Verification items for the finished model (mm, model axes). Face numbers are marked on the shaded views. A direction names the side the tool comes from. Round coordinates to 2 decimals unless told otherwise and drop trailing zeros. Write each loop counter-clockwise with the first axis right and the second up, starting at its lowest first coordinate (ties: lowest second). Pieces come first, ordered by that corner, then holes. Notation, with made-up numbers: M 63.5,88.5 L 106.5,88.5 A13 cw 106.5,103.5 Z; hole C -34.75,24.5 d4. An arc over 180 degrees is marked long. One line per question, with ' | ' between items. Start each with the question number.
Q1. Cross-section at A-A (y = 0). Record the boundary of the cut face in (x, z).
Q2. Tool access check on the marked faces 5 and 6. Record the directions out of +Z, -Z, +X, -X, +Y, -Y that give a thin tool (end or side, any length) a straight path to the whole face; none if there is none.
Q3. Thickness scan on line 1 along Y through (x, z) = (0, -0.65); line 2 along Y through (x, z) = (0, 4.75). Record the ranges inside material, lowest first. Write a range as from..to.
Q4. Cross-section at C-C (z = 9.5). Record the boundary of the cut face in (x, y).
Q5. Release check for a two-part mould opening along Y. For the marked faces 1, 2, 3 and 4 record: released by +Y, released by -Y, zero draft, split by the parting line, or undercut.
Q6. Gauge pin test, flat ends, axial feed: pin 1 (1.5 mm diameter, centred on y = 5.5, z = 0.5, fed in from -X); pin 2 (4 mm diameter, centred on x = -12.5, z = 8.5, fed in from -Y); pin 3 (4 mm diameter, centred on x = -9, z = 2, fed in from +Y); pin 4 (20 mm diameter, centred on x = 0, y = -3, fed in from +Z). Record the tip position at first contact, or that the pin passes through.
from build123d import *

# Parameters (mm, degrees)
F0_R     = 26.15
F1_DEPTH = 13.4
F2_R     = 12.6
F3_DEPTH = 7.4
F4_R     = 8.5
F5_DEPTH = 6
F6_R     = 13.5
F6_R_2   = 8.5
F7_DEPTH = 1
F8_SIZE  = 1


with BuildPart() as f1:
    # F0 (on Top) → F1 (new body)
    with BuildSketch(Plane.XY):
        Circle(F0_R)
    extrude(amount=F1_DEPTH)

    # F2 (on face) → F3 (cut)
    with BuildSketch(Plane.XY.offset(13.4)):
        Circle(F2_R)
    extrude(amount=-F3_DEPTH, mode=Mode.SUBTRACT)

    # F4 (on face) → F5 (cut, through all)
    with BuildSketch(Plane.XY.offset(6)):
        Circle(F4_R)
    extrude(amount=-F5_DEPTH, mode=Mode.SUBTRACT)

    # F6 (on face) → F7 (join)
    with BuildSketch(Plane(origin=(0, 0, 0), x_dir=(1, 0, 0), z_dir=(0, 0, -1))):
        Circle(F6_R)
        Circle(F6_R_2, mode=Mode.SUBTRACT)
    extrude(amount=F7_DEPTH)

    # F8
    f8_edges = [f1.edges().sort_by_distance(p)[0] for p in [
        (-26.15, 0, 13.4),
        (-26.15, 0, 0),
    ]]
    chamfer(f8_edges, length=F8_SIZE)


solid = f1.part
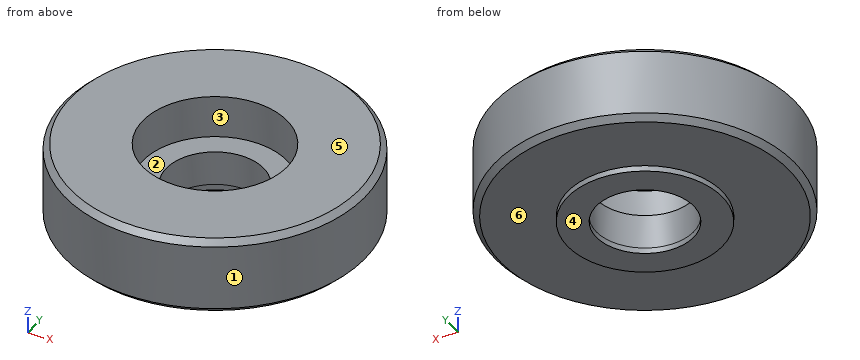
Determined:
1) outline: M -26.15,1 L -25.15,0 L -13.5,0 L -13.5,-1 L -8.5,-1 L -8.5,6 L -12.6,6 L -12.6,13.4 L -25.15,13.4 L -26.15,12.4 Z; M 8.5,-1 L 13.5,-1 L 13.5,0 L 25.15,0 L 26.15,1 L 26.15,12.4 L 25.15,13.4 L 12.6,13.4 L 12.6,6 L 8.5,6 Z
2) face 5: +Z, +X, -X, +Y, -Y | face 6: -Z
3) line 1: y = -13.5..-8.5, 8.5..13.5 | line 2: y = -26.15..-8.5, 8.5..26.15
4) outline: C 0,0 d52.3; hole C 0,0 d25.2
5) face 1: split by the parting line | face 2: undercut | face 3: undercut | face 4: zero draft
6) pin 1: stops at x = -25.68 | pin 2: stops at y = -23.95 | pin 3: stops at y = 25.2 | pin 4: stops at z = 13.4
